```python
from build123d import *

# Parameters (mm, degrees)
SKETCH1_R           = 1.5
BOSS_EXTRUDE1_DEPTH = 42
SKETCH2_R           = 2.75
BOSS_EXTRUDE2_DEPTH = 2.2
ESCALA1_SCALE       = 1.5
ESCALA2_SCALE       = 1.5


with BuildPart() as part:
    # Sketch1 → Boss-Extrude1 (new body)
    with BuildSketch(Plane.XY):
        with Locations(Location((0, 0, 0), (0, 0, 180))):
            Circle(SKETCH1_R)
    extrude(amount=BOSS_EXTRUDE1_DEPTH)

    # Sketch2 → Boss-Extrude2 (add)
    with BuildSketch(Plane(origin=(0, 0, 0), x_dir=(-1, 0, 0), z_dir=(0, 0, -1))):
        Circle(SKETCH2_R)
    extrude(amount=-BOSS_EXTRUDE2_DEPTH)


with BuildPart() as part_1:
    # Escala1: scaled about (0, 0, 0)
    add(part.part.scale(ESCALA1_SCALE))


with BuildPart() as part_2:
    # Escala2: scaled about (0, 0, 0)
    add(part_1.part.scale(ESCALA2_SCALE))


solid = part_2.part
```
Check sheet for the modelled part. Datum: model origin and axes. Units: mm. A direction names the side the tool comes from. Give positions to 0.01 mm unless a question says otherwise; leave off trailing zeros. Order: outer loops, then holes, each group sorted by start corner. A loop starts at its lowest first (then second) coordinate and runs counter-clockwise, first axis right, second up. Notation, with made-up numbers: M 18.25,-21 L 23.25,-21 A24 ccw 23.25,-4 Z; hole C -32,81 d7. An arc over 180 degrees is marked long. Answer in a Markdown table with one row per item.
1) Thickness scan on L1, parallel to Z at x = 1.5, y = 4; L2, parallel to X at y = 1.75, z = 26; L3, parallel to Y at x = 0, z = 44.5 (3 decimals). Record the ranges inside material, lowest first. Write a range as [from, to].
Filled sheet:
| item | result |
|---|---|
| L1 | z = [0, 4.95] |
| L2 | x = [-2.89, 2.89] |
| L3 | y = [-3.375, 3.375] |
2) Gauge pin test, flat ends, axial feed: P1, Ø4, axis at y = -3, z = 59.5, coming from the -X side; P2, Ø6, axis at x = -1, z = 43, coming from the +Y side (3 decimals); P3, Ø4, axis at x = 1.5, y = 4.5, coming from the -Z side; P4, Ø3, axis at y = -2, z = 31, coming from the +X side. Record the tip position at first contact, or that the pin passes through.
Filled sheet:
| item | result |
|---|---|
| P1 | stops at x = -3.22 |
| P2 | stops at y = 3.375 |
| P3 | stops at z = 0 |
| P4 | stops at x = 3.34 |
3) Cross-section at C-C, the plane z = 14. Enter the section's corners in (x, y) (3 decimals), plus the area to 3 significant figures.
Filled sheet:
| item | result |
|---|---|
| outline | C 0,0 d6.75 |
| area | 35.8 mm2 |
4) Cross-section at D-D, the plane x = 5.25. Enter the section's corners in (y, z), plus the area to 3 significant figures.
Filled sheet:
| item | result |
|---|---|
| outline | M -3.27,0 L 3.27,0 L 3.27,4.95 L -3.27,4.95 Z |
| area | 32.4 mm2 |
5) Access from +Z, -Z, +X, -X, +Y, -Y to the whole of each face (thin tool, end or side, straight path). Record for faces 1 (the flat face through (0, 0, 0)), 2 (the flat face through (-3, -3, 4.95)).
Filled sheet:
| item | result |
|---|---|
| face 1 | -Z, +X, -X, +Y, -Y |
| face 2 | +Z |
